CAD build for the part. Positions are in the model's coordinates, mm. A direction names the side the tool comes from. Coordinates: 2 decimals unless noted, no trailing zeros. Loops run counter-clockwise (first coordinate to the right, second up) from the corner with the lowest first, then second, coordinate; pieces in that order, holes last. Notation, with made-up numbers: (32.5, 56.25) -> (44.5, 56.25) arc R5 cw to (44.5, 63.25) -> close; hole circle Ø9 at (43.5, 26). An arc over 180 degrees is marked (long way). Return JSON: item names as keys, results as strings. Group by question number.
(1) Flat gauge pins, fed straight in: pin 1 Ø9 at (x, y) = (2.5, -1.5) entering from +Z; pin 2 Ø1.6 at (x, y) = (13, 3.25) entering from -Z; pin 3 Ø5.5 at (x, y) = (13, -2.5) entering from -Z; pin 4 Ø1.5 at (x, z) = (8.5, 2.5) entering from -Y. Where does each tip first touch, or does it go through?
(2) Saw through at D-D on x = -3.75. Write the cut outline in (y, z).
(3) Saw through at B-B on z = 1.25. Write the cut outline in (x, y).
(4) Probe L1, parallel to Y at x = 12.5, z = 3.75; L2, parallel to X at y = -1, z = 0.5; L3, parallel to Y at x = 11, z = 0.75. List the from-to ranges inside material, lowest first.
(5) Mould opens along X. For faces 4 (the face through (15.4, 8.43, 4.06)), 5 (the face through (-8, 0, 4)), 6 (the face through (-1, -2, 3.8)) say: pulls with the +X half, pulls with the -X half, needs draft (parallel to the pull), parting line crosses it, or undercut.
(6) Saw through at C-C on x = 13. Write the cut outline in (y, z).
(7) Tool access for faces 1 (the face through (-7.65, -2.18, 4.06)), 2 (the face through (13, 3, 4.2)), 3 (the face through (10.502, -3.14, 8.74)): list every direction of +Z, -Z, +X, -X, +Y, -Y with a clear straight run to the whole face (end or side of a thin tool).
(8) Saw through at A-A on y = 0. Write the cut outline in (x, z), then the cut area to 3 significant figures.
```python
from build123d import *

# Parameters (mm, degrees)
ESQUISSE1_W             = 24
ESQUISSE1_H             = 18
BOSS_EXTRU_1_DEPTH      = 8
ESQUISSE2_R             = 2.2
ENL_V_MAT_EXTRU_1_DEPTH = 9
ESQUISSE3_R             = 4
ENL_V_MAT_EXTRU_2_DEPTH = 4.2
ESQUISSE4_R             = 1
ENL_V_MAT_EXTRU_3_DEPTH = 9
ESQUISSE5_R             = 2.6
ENL_V_MAT_EXTRU_6_DEPTH = 4.2
ESQUISSE6_R             = 1.7
BOSS_EXTRU_2_DEPTH      = 1
CHANFREIN1_SIZE         = 18
CHANFREIN1_SIZE2        = 6.551464217
CHANFREIN1_PART_2_SIZE  = 18
CHANFREIN1_PART_2_SIZE2 = 6.551464217
CONG_1_R                = 2
ESQUISSE7_R             = 2.5
ESQUISSE7_R_2           = 1
BOSS_EXTRU_3_DEPTH      = 1.5


with BuildPart() as part:
    # Esquisse1 → Boss.-Extru.1 (new body)
    with BuildSketch(Plane.XY):
        with Locations((4, 0)):
            Rectangle(ESQUISSE1_W, ESQUISSE1_H)
    extrude(amount=BOSS_EXTRU_1_DEPTH)

    # Esquisse2 → Enlèv. mat.-Extru.1 (cut, through all)
    with BuildSketch(Plane.XY.offset(8)):
        with Locations((-3, 0)):
            Circle(ESQUISSE2_R)
    extrude(amount=-ENL_V_MAT_EXTRU_1_DEPTH, mode=Mode.SUBTRACT)

    # Esquisse3 → Enlèv. mat.-Extru.2 (cut)
    with BuildSketch(Plane.XY.offset(8)):
        with Locations((-3, 0)):
            Circle(ESQUISSE3_R)
    extrude(amount=-ENL_V_MAT_EXTRU_2_DEPTH, mode=Mode.SUBTRACT)

    # Esquisse4 → Enlèv. mat.-Extru.3 (cut, through all)
    with BuildSketch(Plane.XY.offset(8)):
        with Locations((13, 3.25)):
            Circle(ESQUISSE4_R)
        with Locations((13, -3.25)):
            Circle(ESQUISSE4_R)
    extrude(amount=-ENL_V_MAT_EXTRU_3_DEPTH, mode=Mode.SUBTRACT)

    # Esquisse5 → Enlèv. mat.-Extru.6 (cut)
    with BuildSketch(Plane(origin=(0, 0, 0), x_dir=(-1, 0, 0), z_dir=(0, 0, -1))):
        with Locations((-13, 3.25)):
            Circle(ESQUISSE5_R)
        with Locations((-13, -3.25)):
            Circle(ESQUISSE5_R)
    extrude(amount=-ENL_V_MAT_EXTRU_6_DEPTH, mode=Mode.SUBTRACT)

    # Esquisse6 → Boss.-Extru.2 (add)
    with BuildSketch(Plane(origin=(0, 0, 4.2), x_dir=(-1, 0, 0), z_dir=(0, 0, -1))):
        with Locations((-13, 3.25)):
            Circle(ESQUISSE6_R)
        with Locations((-13, -3.25)):
            Circle(ESQUISSE6_R)
    extrude(amount=-BOSS_EXTRU_2_DEPTH)

    # Chanfrein1
    chanfrein1_edges = [part.edges().sort_by_distance(p)[0] for p in [
        (-8, 9, 4),
    ]]
    chanfrein1_side = [part.faces().sort_by_distance(p)[0] for p in [
        (4, 9, 4),
    ]]
    chamfer(chanfrein1_edges, length=CHANFREIN1_SIZE, length2=CHANFREIN1_SIZE2, reference=chanfrein1_side[0])

    # Chanfrein1 part 2
    chanfrein1_part_2_edges = [part.edges().sort_by_distance(p)[0] for p in [
        (-8, -9, 4),
    ]]
    chanfrein1_part_2_side = [part.faces().sort_by_distance(p)[0] for p in [
        (4, -9, 4),
    ]]
    chamfer(chanfrein1_part_2_edges, length=CHANFREIN1_PART_2_SIZE, length2=CHANFREIN1_PART_2_SIZE2, reference=chanfrein1_part_2_side[0])

    # Congé1
    cong_1_edges = [part.edges().sort_by_distance(p)[0] for p in [
        (10, -9, 4),
        (-8, 2.448535783, 4),
        (-8, -2.448535783, 4),
        (10, 9, 4),
        (16, 9, 4),
        (16, -9, 4),
    ]]
    fillet(cong_1_edges, radius=CONG_1_R)

    # Esquisse7 → Boss.-Extru.3 (add)
    with BuildSketch(Plane.XY.offset(8)):
        with Locations((13, -3.25)):
            Circle(ESQUISSE7_R)
        with Locations((13, -3.25)):
            Circle(ESQUISSE7_R_2, mode=Mode.SUBTRACT)
        with Locations((13, 3.25)):
            Circle(ESQUISSE7_R)
        with Locations((13, 3.25)):
            Circle(ESQUISSE7_R_2, mode=Mode.SUBTRACT)
    extrude(amount=BOSS_EXTRU_3_DEPTH)


solid = part.part
```
Geometry results:
{
 "1": {"pin 1": "z = 8", "pin 2": "z = 4.2", "pin 3": "z = 0", "pin 4": "y = -8.73"},
 "2": {"outline": "(-4, 0) -> (-2.07, 0) -> (-2.07, 3.8) -> (-3.93, 3.8) -> (-3.93, 8) -> (-4, 8) -> close; (2.07, 0) -> (4, 0) -> (4, 8) -> (3.93, 8) -> (3.93, 3.8) -> (2.07, 3.8) -> close"},
 "3": {"outline": "(-8, -1.05) arc R2 ccw to (-6.68, -2.93) -> (9.67, -8.88) arc R2 ccw to (10.35, -9) -> (14, -9) arc R2 ccw to (16, -7) -> (16, 7) arc R2 ccw to (14, 9) -> (10.35, 9) arc R2 ccw to (9.67, 8.88) -> (-6.68, 2.93) arc R2 ccw to (-8, 1.05) -> close; hole circle Ø4.4 at (-3, 0); hole circle Ø5.2 at (13, -3.25); hole circle Ø5.2 at (13, 3.25)"},
 "4": {"L1": "-9 to -5.8, -0.7 to 0.7, 5.8 to 9", "L2": "-8 to -4.96, -1.04 to 11.7, 14.3 to 16", "L3": "-9 to -4.91, -1.59 to 1.59, 4.91 to 9"},
 "5": {"face 4": "pulls with the +X half", "face 5": "pulls with the -X half", "face 6": "undercut"},
 "6": {"outline": "(-9, 0) -> (-5.85, 0) -> (-5.85, 4.2) -> (-0.65, 4.2) -> (-0.65, 0) -> (0.65, 0) -> (0.65, 4.2) -> (5.85, 4.2) -> (5.85, 0) -> (9, 0) -> (9, 8) -> (5.75, 8) -> (5.75, 9.5) -> (4.25, 9.5) -> (4.25, 5.2) -> (2.25, 5.2) -> (2.25, 9.5) -> (0.75, 9.5) -> (0.75, 8) -> (-0.75, 8) -> (-0.75, 9.5) -> (-2.25, 9.5) -> (-2.25, 5.2) -> (-4.25, 5.2) -> (-4.25, 9.5) -> (-5.75, 9.5) -> (-5.75, 8) -> (-9, 8) -> close"},
 "7": {"face 1": "+Z, -Z, -X, -Y", "face 2": "-Z", "face 3": "+Z"},
 "8": {"outline": "(-8, 0) -> (-5.2, 0) -> (-5.2, 3.8) -> (-7, 3.8) -> (-7, 8) -> (-8, 8) -> close; (-0.8, 0) -> (16, 0) -> (16, 8) -> (1, 8) -> (1, 3.8) -> (-0.8, 3.8) -> close", "area": "142 mm²"}
}
